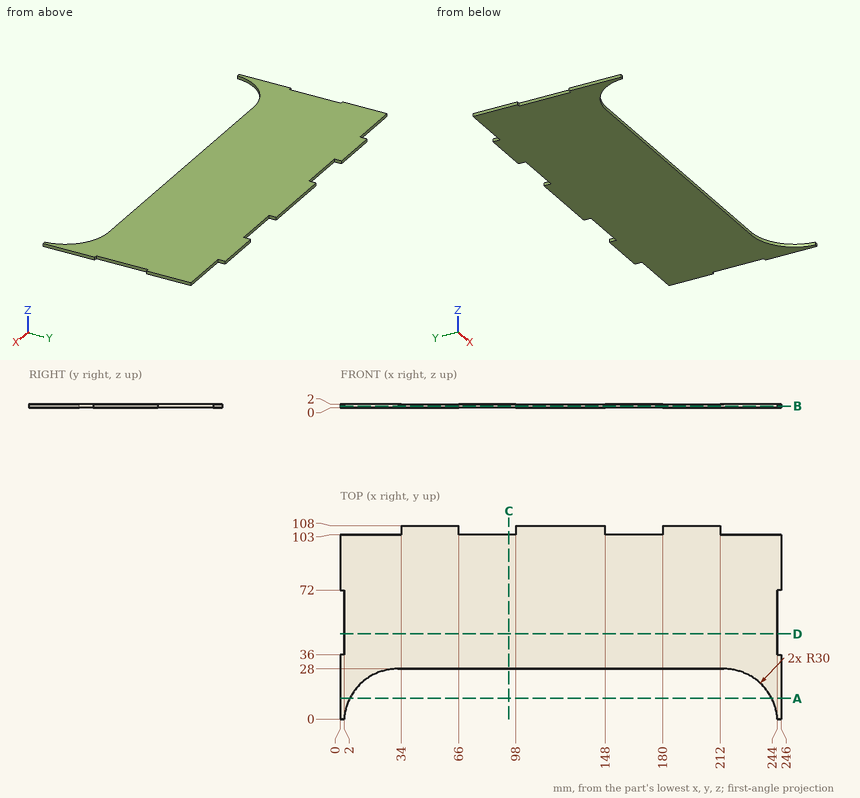
Geometry: see drawing. Coordinates: mm, zero at the bounding-box minimum. Round coordinates to 2 decimals unless told otherwise and drop trailing zeros. Write each loop counter-clockwise with the first axis right and the second up, starting at its lowest first coordinate (ties: lowest second). Pieces come first, ordered by that corner, then holes. Notation, with made-up numbers: M 28.25,74 L 82.25,74 A19 cw 82.25,81 Z; hole C 38.25,71.5 d8. An arc over 180 degrees is marked long. Answer as a JSON object with one key per item and string values. Group by question number.
(1) Section query C-C on x = 94. Output: boundary loops of the cut face in (y, z).
(2) First-contact query: pin 1 (1 mm diameter, centred on x = 20, z = 1.5, fed in from +Y); pin 2 (1 mm diameter, centred on y = 105, z = 0.5, fed in from -X); pin 3 (1 mm diameter, centred on y = 46.5, z = 0.5, fed in from +X). Flat tips, straight axial feed; report the tip coordinate or a pass-through.
(3) Ray query, line 1 (Y direction, x = 139.5, z = 1.15); line 2 (Y direction, x = 172.5, z = 0.1); line 3 (X direction, y = 20, z = 0.15). Return the intervals inside material, ascending. Write a range as [from, to].
(4) Section query A-A on y = 11.5. Output: boundary loops of the cut face in (x, z).
(5) Section query D-D on y = 47.5. Output: boundary loops of the cut face in (x, z).
(6) Section query B-B on z = 0.8. Output: boundary loops of the cut face in (x, y).
Computed values:
{
 "1": {"outline": "M 28,0 L 103,0 L 103,2 L 28,2 Z"},
 "2": {"pin 1": "y = 103", "pin 2": "x = 34", "pin 3": "x = 244"},
 "3": {"line 1": "[28, 108]", "line 2": "[28, 103]", "line 3": "[0, 11.6], [234.4, 246]"},
 "4": {"outline": "M 0,0 L 5.21,0 L 5.21,2 L 0,2 Z; M 240.79,0 L 246,0 L 246,2 L 240.79,2 Z"},
 "5": {"outline": "M 2,0 L 244,0 L 244,2 L 2,2 Z"},
 "6": {"outline": "M 0,0 L 2.07,0 A30 cw 32,28 L 214,28 A30 cw 243.93,0 L 246,0 L 246,36 L 244,36 L 244,72 L 246,72 L 246,103 L 212,103 L 212,108 L 180,108 L 180,103 L 148,103 L 148,108 L 98,108 L 98,103 L 66,103 L 66,108 L 34,108 L 34,103 L 0,103 L 0,72 L 2,72 L 2,36 L 0,36 Z"}
}
